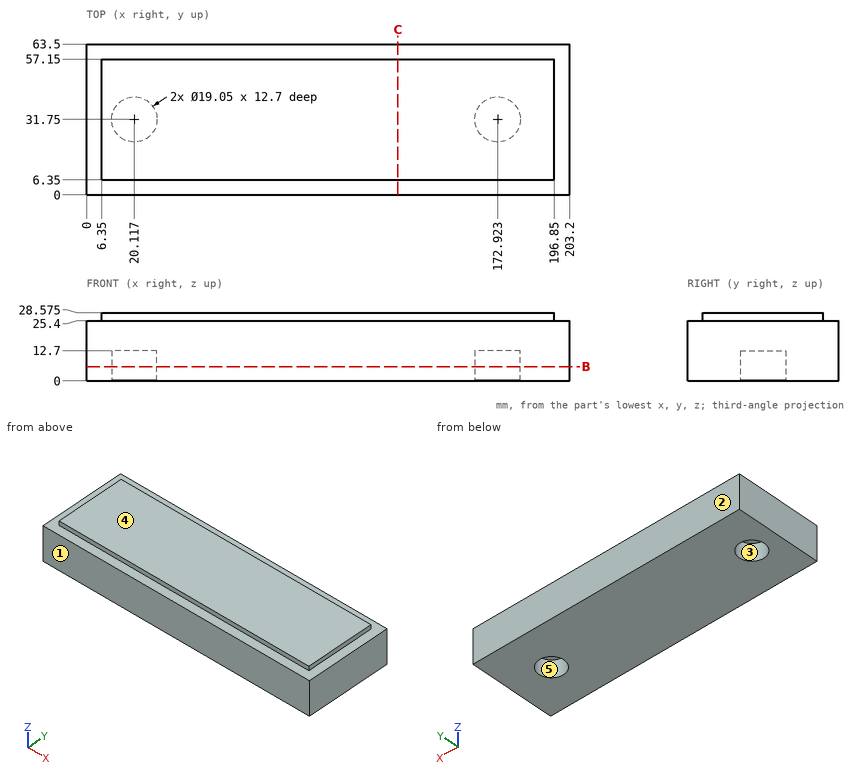
The figure shows three views and two pictorial views of one solid part (mm, origin at its lowest corner). Answer the questions. A direction names the side the tool comes from. Give positions to 0.01 mm unless a question says otherwise; leave off trailing zeros. Write each loop counter-clockwise with the first axis right and the second up, starting at its lowest first coordinate (ties: lowest second). Pieces come first, ordered by that corner, then holes. Notation, with made-up numbers: (17, 23.5) - (42, 23.5) arc R27 ccw to (42, 57.5) - close; hole circle Ø9 at (-23, 50.25). An arc over 180 degrees is marked (long way). Return JSON: item names as keys, results as strings.
Q1. For a pull along Y with two mould halves and no side action, classify the marked faces 1, 2 and 3 as released by +Y, released by -Y, zero draft, split by the parting line, or undercut.
Reply:
{"face 1": "released by -Y", "face 2": "released by +Y", "face 3": "undercut"}
Q2. A cutting plane is placed at B-B, the plane z = 6. Count the separate pieces of the cut face and the enclosed holes in it, and give its area (3 significant figures).
Reply:
{"separate pieces": "1", "enclosed holes": "2", "area": "12,300 mm²"}
Q3. Consider line 1 along X through (y, z) = (31.75, 9); line 2 along X through (y, z) = (27, 7.5); line 3 along Z through (x, y) = (24.5, 57.5). Determine where each line is inside the solid, lowest interval first. Write a range as [from, to].
Reply:
{"line 1": "[0, 10.59], [29.64, 163.4], [182.45, 203.2]", "line 2": "[0, 11.86], [28.37, 164.67], [181.18, 203.2]", "line 3": "[0, 25.4]"}
Q4. A cutting plane is placed at C-C, the plane x = 131. Determine the outline of the cut face in (y, z) (3 decimals).
Reply:
{"outline": "(0, 0) - (63.5, 0) - (63.5, 25.4) - (57.15, 25.4) - (57.15, 28.575) - (6.35, 28.575) - (6.35, 25.4) - (0, 25.4) - close"}
Q5. Given P1, Ø1, axis at x = 149, z = 27.5, coming from the -Y side; P2, Ø3.5, axis at x = 82.5, z = 27, coming from the +Y side; P3, Ø5.5, axis at x = 22.5, y = 29.5, coming from the -Z side; P4, Ø2.5, axis at y = 39.5, z = 27, coming from the +X side, each flat-ended and moving along its own axis, determine where each tip first touches the part or whether it passes through.
Reply:
{"P1": "y = 6.35", "P2": "y = 63.5", "P3": "z = 12.7", "P4": "x = 196.85"}
Q6. For the marked faces 4 and 5, determine the directions among +Z, -Z, +X, -X, +Y, -Y from which every point of the face is accessible in a straight line to the end or side of a thin tool.
Reply:
{"face 4": "+Z, +X, -X, +Y, -Y", "face 5": "-Z"}
